Input: dimensioned drawing with shaded views. Units: mm. Origin: part minimum x, y, z. Coordinates: 2 decimals unless noted, no trailing zeros. Order: outer loops, then holes, each group sorted by start corner. A loop starts at its lowest first (then second) coordinate and runs counter-clockwise, first axis right, second up.
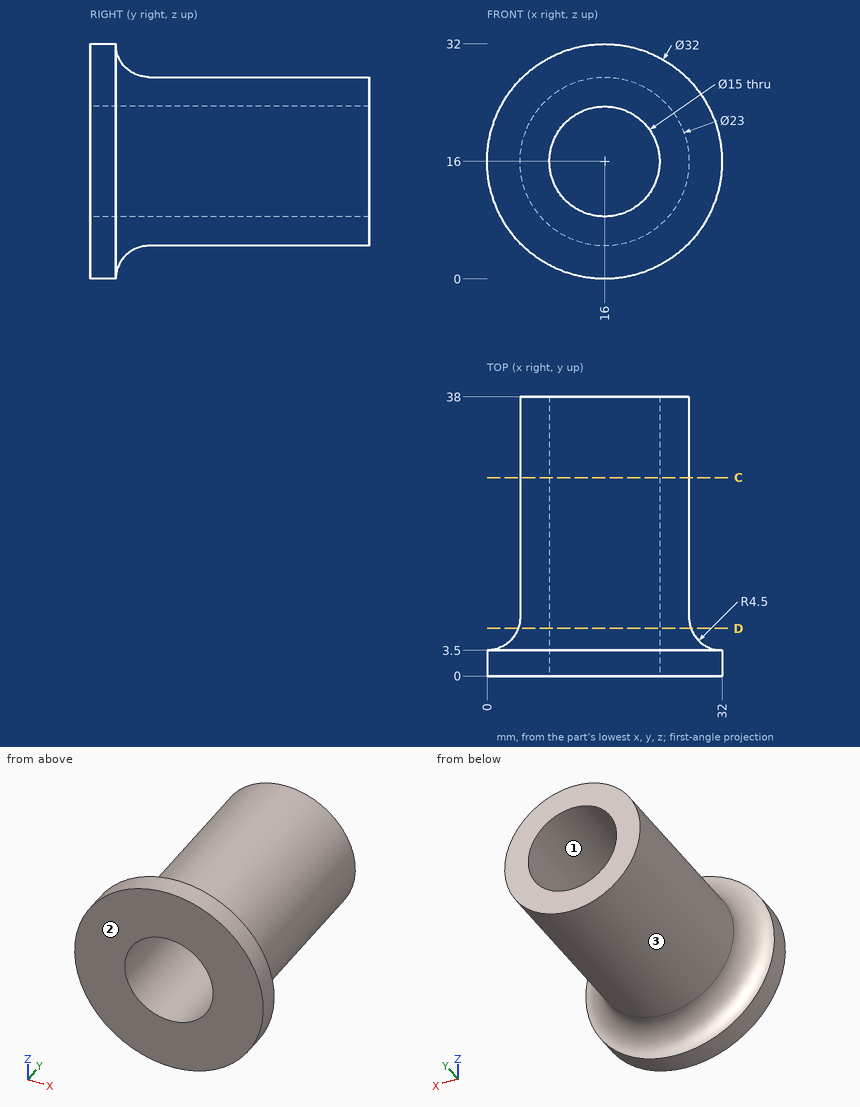
1. Pin query (flat end, axial travel): P1, Ø12, axis at y = 18, z = 24.5, coming from the -X side (3 decimals); P2, Ø13.5, axis at x = 16, z = 16, coming from the +Y side; P3, Ø1, axis at x = 9, y = 10, coming from the -Z side; P4, Ø2, axis at x = 19.5, y = 30, coming from the -Z side (3 decimals). Return the tip coordinate at first contact, or that it passes through.
Findings:
P1: stops at x = 4.775
P2: passes through
P3: stops at z = 6.51
P4: stops at z = 4.775
2. Section query C-C on y = 27. Return loops of the section in (x, z), plus the area to 3 significant figures.
Findings:
outline: circle Ø23 at (16, 16); hole circle Ø15 at (16, 16)
area: 239 mm2
3. Section query D-D on y = 6.5. Return loops of the section in (x, z).
Findings:
outline: circle Ø23.51 at (16, 16); hole circle Ø15 at (16, 16)
4. Draft query along X for the marked faces 1, 2 and 3. Return one class per face: released by +X, released by -X, zero draft, split by the parting line, or undercut.
Findings:
face 1: undercut
face 2: zero draft
face 3: split by the parting line
5. Ray query, line 1 (X direction, y = 23, z = 16); line 2 (Z direction, x = 14, y = 35) (1 decimal); line 3 (X direction, y = 3, z = 9.5). Return the intervals inside material, ascending.
Findings:
line 1: x = 4.5 to 8.5, 23.5 to 27.5
line 2: z = 4.7 to 8.8, 23.2 to 27.3
line 3: x = 1.38 to 12.26, 19.74 to 30.62
